Input: dimensioned drawing with shaded views. Units: mm. Origin: part minimum x, y, z. A direction names the side the tool comes from. Give positions to 0.01 mm unless a question says otherwise; leave off trailing zeros. Loops run counter-clockwise (first coordinate to the right, second up) from the corner with the lowest first, then second, coordinate; pieces in that order, holes last. Notation, with made-up numbers: (57.25, 63.5) -> (75.25, 63.5) arc R21 cw to (75.25, 94.5) -> close; hole circle Ø2 at (77.25, 17). An arc over 180 degrees is marked (long way). One line per question, with ' | ' between items. Start each with the question number.
Item 1: Section D-D on y = 27.5. Return loops of the section in (x, z), then the cut area to 3 significant figures.
Item 2: Mould query, pull axis Z, two halves, no side actions, for the marked faces 4, 5, 6 and 7. Classes: released by +Z, released by -Z, zero draft, split by the parting line, or undercut.
Item 3: Material intervals for line 1 along Y through (x, z) = (34.5, 40); line 2 along Y through (x, z) = (70, 99.5); line 3 along Y through (x, z) = (25, 64.5), sorted ascending. Write a range as [from, to].
Item 4: Set-up query: the marked faces 1, 2 and 3. Return all of +Z, -Z, +X, -X, +Y, -Y with unobstructed straight access to the full face (end or side cutting, diameter ignored); none if empty.
Item 5: Pin query (flat end, axial travel): P1, Ø15, axis at x = 14.5, z = 21, coming from the -Y side; P2, Ø20, axis at x = 64, z = 37, coming from the -Y side; P3, Ø15, axis at x = 87, y = 9.5, coming from the +Z side. Return the tip coordinate at first contact, or that it passes through.
Item 6: Section C-C on y = 70. Return loops of the section in (x, z), then the cut area to 3 significant figures.
Item 7: Section A-A on x = 35. Return loops of the section in (y, z).
Item 8: Section B-B on z = 76. Return loops of the section in (x, y).
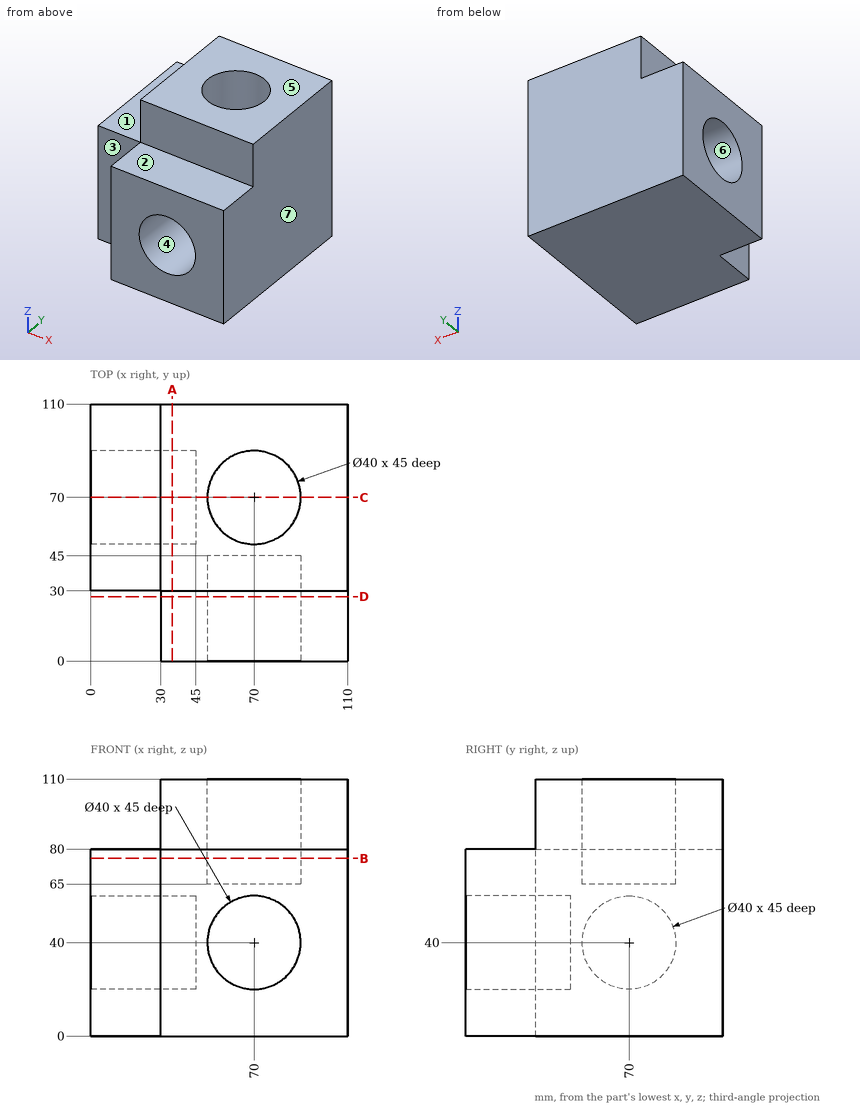
Result sheet:
1) outline: (30, 0) -> (110, 0) -> (110, 80) -> (30, 80) -> close; hole circle Ø40 at (70, 40) | area: 5,140 mm²
2) face 4: undercut | face 5: released by +Z | face 6: undercut | face 7: zero draft
3) line 1: y = [0, 50], [90, 110] | line 2: y = [30, 50], [90, 110] | line 3: y = [30, 110]
4) face 1: +Z, -X, +Y, -Y | face 2: +Z, +X, -X, -Y | face 3: +Z, -Z, -X, -Y
5) P1: stops at y = 30 | P2: stops at y = 45 | P3: stops at z = 80
6) outline: (0, 0) -> (110, 0) -> (110, 110) -> (90, 110) -> (90, 65) -> (50, 65) -> (50, 110) -> (30, 110) -> (30, 80) -> (0, 80) -> (0, 60) -> (45, 60) -> (45, 20) -> (0, 20) -> close | area: 7,600 mm²
7) outline: (0, 0) -> (110, 0) -> (110, 110) -> (30, 110) -> (30, 80) -> (0, 80) -> close; hole circle Ø40 at (70, 40)
8) outline: (0, 30) -> (30, 30) -> (30, 0) -> (110, 0) -> (110, 110) -> (0, 110) -> close; hole circle Ø40 at (70, 70)
